Could you check a few things on this model? Use its own coordinates, in mm. Face numbers are marked on the shaded views. A direction names the side the tool comes from. Give positions to 0.01 mm unless a question says otherwise; leave off trailing zeros. Order: outer loops, then holes, each group sorted by start corner. A loop starts at its lowest first (then second) coordinate and runs counter-clockwise, first axis right, second up. Notation, with made-up numbers: (89.25, -38) -> (133.25, -38) arc R38 ccw to (133.25, 1) -> close; hole circle Ø6 at (33.5, -1.75). An arc over 180 degrees is marked (long way). Write each question's results on one line, items separated by ' | '.
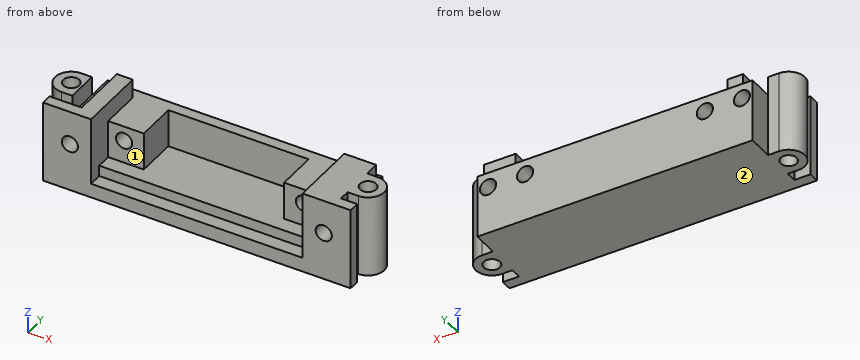
```python
from build123d import *

# Parameters (mm, degrees)
SKETCH_W        = 51
SKETCH_H        = 20
PAD_DEPTH       = 15.15
POCKET_DEPTH    = 10.5
SKETCH002_W     = 39.2
SKETCH002_H     = 2.5
POCKET001_DEPTH = 2
SKETCH011_W     = 51
SKETCH011_H     = 5.25
POCKET002_DEPTH = 15.151
SKETCH012_W     = 3
SKETCH012_H     = 15.15
PAD005_DEPTH    = 2
SKETCH013_R     = 1.5
POCKET003_DEPTH = 14.751
SKETCH014_W     = 39.2
SKETCH014_H     = 3.5
POCKET004_DEPTH = 7.5
SKETCH015_W     = 2
SKETCH015_H     = 3.5
POCKET005_DEPTH = 54.001
SKETCH016_W     = 2.95
SKETCH016_H     = 3.5
POCKET006_DEPTH = 10.75
SKETCH017_R     = 1.5
PAD006_DEPTH    = 15.15


with BuildPart() as part:
    # Sketch → Pad (new body)
    with BuildSketch(Plane.XY):
        Rectangle(SKETCH_W, SKETCH_H)
    extrude(amount=PAD_DEPTH)

    # Sketch001 (on Face6 of Pad) → Pocket (cut)
    with BuildSketch(Plane.XY.offset(15.15)):
        Polygon((-19.6, -10), (19.6, -10), (19.6, -4.75), (13, -4.75), (13, 2.75), (-13, 2.75), (-13, -4.75), (-19.6, -4.75), align=None)
    extrude(amount=-POCKET_DEPTH, mode=Mode.SUBTRACT)

    # Sketch002 (on Face14 of Pocket) → Pocket001 (cut)
    with BuildSketch(Plane.XY.offset(4.65)):
        with Locations((0, -8.75)):
            Rectangle(SKETCH002_W, SKETCH002_H)
    extrude(amount=-POCKET001_DEPTH, mode=Mode.SUBTRACT)

    # Sketch011 (on Face5 of Pocket001) → Pocket002 (cut, through all)
    with BuildSketch(Plane.XY.offset(15.15)):
        with Locations((0, 7.375)):
            Rectangle(SKETCH011_W, SKETCH011_H)
    extrude(amount=-POCKET002_DEPTH, mode=Mode.SUBTRACT)

    # Sketch012 (on Face5 of Pocket002) → Pad005 (join)
    with BuildSketch(Plane.XZ.offset(10)):
        with Locations((-27, 7.575)):
            Rectangle(SKETCH012_W, SKETCH012_H)
        with Locations((27, 7.575)):
            Rectangle(SKETCH012_W, SKETCH012_H)
    extrude(amount=-PAD005_DEPTH)

    # Sketch013 (on Face8 of Pad005) → Pocket003 (cut, through all)
    with BuildSketch(Plane.XZ.offset(10)):
        with Locations((-23.52, 8.9)):
            Circle(SKETCH013_R)
        with Locations((-16.66, 8.9)):
            Circle(SKETCH013_R)
        with Locations((16.66, 8.9)):
            Circle(SKETCH013_R)
        with Locations((23.52, 8.9)):
            Circle(SKETCH013_R)
    extrude(amount=-POCKET003_DEPTH, mode=Mode.SUBTRACT)

    # Sketch014 (on Face20 of Pocket003) → Pocket004 (cut)
    with BuildSketch(Plane.XZ.offset(4.75)):
        with Locations((0, 13.4)):
            Rectangle(SKETCH014_W, SKETCH014_H)
    extrude(amount=-POCKET004_DEPTH, mode=Mode.SUBTRACT)

    # Sketch015 (on Face1 of Pocket004) → Pocket005 (cut, through all)
    with BuildSketch(Plane(origin=(-25.5, 0, 0), x_dir=(0, -1, 0), z_dir=(-1, 0, 0))):
        with Locations((-3.75, 13.4)):
            Rectangle(SKETCH015_W, SKETCH015_H)
    extrude(amount=-POCKET005_DEPTH, mode=Mode.SUBTRACT)

    # Sketch016 (on Face5 of Pocket005) → Pocket006 (cut)
    with BuildSketch(Plane(origin=(0, 2.75, 0), x_dir=(-1, 0, 0), z_dir=(0, 1, 0))):
        with Locations((24.025, 13.4)):
            Rectangle(SKETCH016_W, SKETCH016_H)
    extrude(amount=-POCKET006_DEPTH, mode=Mode.SUBTRACT)

    # Sketch017 (on Face25 of Pocket006) → Pad006 (join)
    with BuildSketch(Plane.XY.offset(15.15)):
        with BuildLine():
            Line((-25.5, 0), (-25.5, -6))
            Line((-27.5, -6), (-25.5, -6))
            ThreePointArc((-27.5, 0), (-30.5, -3), (-27.5, -6))
            Line((-27.5, 0), (-25.5, 0))
        make_face()
        with Locations((-27.5, -3)):
            Circle(SKETCH017_R, mode=Mode.SUBTRACT)
        with BuildLine():
            Line((25.5, 0), (25.5, -6))
            Line((25.5, -6), (27.5, -6))
            ThreePointArc((27.5, -6), (30.5, -3), (27.5, 0))
            Line((25.5, 0), (27.5, 0))
        make_face()
        with Locations((27.5, -3)):
            Circle(SKETCH017_R, mode=Mode.SUBTRACT)
    extrude(amount=-PAD006_DEPTH)


solid = part.part
```
Q1. I'm going to push flat-ended pins straight in: pin 1 Ø1.8 at (x, z) = (21.5, 13.5) entering from +Y; pin 2 Ø0.9 at (x, z) = (27, 11) entering from +Y; pin 3 Ø6 at (x, y) = (-7.5, -3) entering from +Z. Where does each tip first touch, or does it pass through?
Here are the results:
pin 1: stops at y = 2.75 | pin 2: stops at y = 0 | pin 3: stops at z = 4.65
Q2. Suppose I cut it at A-A on y = -3. Please give me the cut outline in (x, z).
Here are the results:
outline: (-30.5, 0) -> (-29, 0) -> (-29, 15.15) -> (-30.5, 15.15) -> close; (-26, 0) -> (26, 0) -> (26, 15.15) -> (19.6, 15.15) -> (19.6, 11.65) -> (13, 11.65) -> (13, 4.65) -> (-13, 4.65) -> (-13, 11.65) -> (-19.6, 11.65) -> (-19.6, 15.15) -> (-22.55, 15.15) -> (-22.55, 11.65) -> (-25.5, 11.65) -> (-25.5, 15.15) -> (-26, 15.15) -> close; (29, 0) -> (30.5, 0) -> (30.5, 15.15) -> (29, 15.15) -> close; hole circle Ø3 at (-23.52, 8.9); hole circle Ø3 at (-16.66, 8.9); hole circle Ø3 at (16.66, 8.9); hole circle Ø3 at (23.52, 8.9)
Q3. Suppose I cut it at C-C on x = 16.66. Please give me the cut outline in (y, z).
Here are the results:
outline: (-10, 0) -> (4.75, 0) -> (4.75, 7.4) -> (-4.75, 7.4) -> (-4.75, 4.65) -> (-7.5, 4.65) -> (-7.5, 2.65) -> (-10, 2.65) -> close; (-4.75, 10.4) -> (4.75, 10.4) -> (4.75, 11.65) -> (-4.75, 11.65) -> close
Q4. Suppose I cut it at B-B on z = 13.75. Please give me the cut outline in (x, y).
Here are the results:
outline: (-28.5, -10) -> (-19.6, -10) -> (-19.6, 2.75) -> (-22.55, 2.75) -> (-22.55, -8) -> (-28.5, -8) -> close; (-27.5, -6) -> (-25.5, -6) -> (-25.5, 0) -> (-27.5, 0) arc R3 ccw to start; (19.6, -10) -> (28.5, -10) -> (28.5, -8) -> (25.5, -8) -> (25.5, -6) -> (27.5, -6) arc R3 ccw to (27.5, 0) -> (25.5, 0) -> (25.5, 2.75) -> (19.6, 2.75) -> close; hole circle Ø3 at (-27.5, -3); hole circle Ø3 at (27.5, -3)
Q5. Suppose I cut it at D-D on y = -9. Please give me the cut outline in (x, z).
Here are the results:
outline: (-28.5, 0) -> (28.5, 0) -> (28.5, 15.15) -> (19.6, 15.15) -> (19.6, 2.65) -> (-19.6, 2.65) -> (-19.6, 15.15) -> (-28.5, 15.15) -> close; hole circle Ø3 at (-23.52, 8.9); hole circle Ø3 at (23.52, 8.9)
Q6. I need wall thicknesses on line 1 along Y through (x, z) = (27.5, 7); line 2 along X through (y, z) = (1.5, 9); line 3 along Z through (x, y) = (-23.52, -6.25). Which ranges of each line are inside material? Lowest first, please.
Here are the results:
line 1: y = -10 to -8, -6 to -4.5, -1.5 to 0 | line 2: x = -25.5 to -25.02, -22.02 to -18.16, -15.16 to -13, 13 to 15.16, 18.16 to 22.02, 25.02 to 25.5 | line 3: z = 0 to 7.4, 10.4 to 11.65
Q7. For the marked faces 1 and 2, which set-ups out of +Z, -Z, +X, -X, +Y, -Y let a thin tool reach every point of the face, with its end or its side?
Here are the results:
face 1: +Z, -Y | face 2: -Z, +X, -X, +Y, -Y
